from build123d import *

# Parameters (mm, degrees)
SKETCH_1_W          = 228
SKETCH_1_H          = 84
SKETCH_1_R          = 2.15
EXTRUDE_1_DEPTH     = 1
SKETCH_3_R          = 1.7
SKETCH_3_R_2        = 1.6
SKETCH_3_R_3        = 4
CUT_EXTRUDE_1_DEPTH = 10
SKETCH_4_R          = 3.5
SKETCH_4_R_2        = 1.6
CUT_EXTRUDE_2_DEPTH = 1
SKETCH_5_R          = 1.7
SKETCH_5_R_2        = 3
CUT_EXTRUDE_3_DEPTH = 10


with BuildPart() as part:
    # Эскиз1 → Вытянуть1 (new body)
    with BuildSketch(Plane.XY):
        Rectangle(SKETCH_1_W, SKETCH_1_H)
        with Locations((107, 32)):
            Circle(SKETCH_1_R, mode=Mode.SUBTRACT)
        with Locations(Location((-107, 32, 0), (0, 0, 180))):
            Circle(SKETCH_1_R, mode=Mode.SUBTRACT)
        with Locations((-107, -32)):
            Circle(SKETCH_1_R, mode=Mode.SUBTRACT)
        with Locations(Location((107, -32, 0), (0, 0, 180))):
            Circle(SKETCH_1_R, mode=Mode.SUBTRACT)
    extrude(amount=EXTRUDE_1_DEPTH)

    # Эскиз3 → Вырез-Вытянуть1 (cut)
    with BuildSketch(Plane.XY.offset(1)):
        with Locations((37, -22)):
            Circle(SKETCH_3_R)
        with Locations((84, -22)):
            Circle(SKETCH_3_R)
        with Locations((38.5, 17)):
            Circle(SKETCH_3_R_2)
        with Locations((82.5, 17)):
            Circle(SKETCH_3_R_2)
        with Locations((51.5, 22)):
            Circle(SKETCH_3_R_3)
        with Locations((69.5, 22)):
            Circle(SKETCH_3_R_3)
        with BuildLine():
            Line((40.14870942, -25.864196381), (40.875982147, -17.864196381))
            ThreePointArc((40.875982147, -17.864196381), (41.358314525, -16.892366164), (42.369821957, -16.5))
            Line((42.369821957, -16.5), (78.630178043, -16.5))
            ThreePointArc((78.630178043, -16.5), (79.641685475, -16.892366164), (80.124017853, -17.864196381))
            Line((80.124017853, -17.864196381), (80.85129058, -25.864196381))
            ThreePointArc((80.85129058, -25.864196381), (80.465084606, -27.011507432), (79.35745077, -27.5))
            Line((79.35745077, -27.5), (41.64254923, -27.5))
            ThreePointArc((41.64254923, -27.5), (40.534915394, -27.011507432), (40.14870942, -25.864196381))
        make_face()
    extrude(amount=-CUT_EXTRUDE_1_DEPTH, mode=Mode.SUBTRACT)

    # Эскиз4 → Вырез-Вытянуть2 (cut)
    with BuildSketch(Plane.XY.offset(1)):
        with Locations((-108, 9)):
            Circle(SKETCH_4_R)
        with Locations((-102, -15)):
            Circle(SKETCH_4_R_2)
        with Locations((-37, -15)):
            Circle(SKETCH_4_R_2)
        with Locations((-26, -15)):
            Circle(SKETCH_4_R_2)
        with Locations((23, -15)):
            Circle(SKETCH_4_R_2)
        with BuildLine():
            Line((-84.5, -9.5), (-54.5, -9.5))
            ThreePointArc((-54.5, -9.5), (-47, -17), (-54.5, -24.5))
            Line((-54.5, -24.5), (-84.5, -24.5))
            ThreePointArc((-84.5, -24.5), (-92, -17), (-84.5, -9.5))
        make_face()
        with BuildLine():
            Line((-9, -9.5), (6, -9.5))
            ThreePointArc((6, -9.5), (13.5, -17), (6, -24.5))
            Line((6, -24.5), (-9, -24.5))
            ThreePointArc((-9, -24.5), (-16.5, -17), (-9, -9.5))
        make_face()
    extrude(amount=-CUT_EXTRUDE_2_DEPTH, mode=Mode.SUBTRACT)

    # Эскиз5 → Вырез-Вытянуть3 (cut)
    with BuildSketch(Plane.XY.offset(1)):
        with Locations((-84, 22)):
            Circle(SKETCH_5_R)
        with Locations((6, 22)):
            Circle(SKETCH_5_R)
        with Locations((-4, 22)):
            Circle(SKETCH_5_R_2)
        with Locations((-14, 22)):
            Circle(SKETCH_5_R_2)
        with Locations((-24, 22)):
            Circle(SKETCH_5_R_2)
        with Locations((-34, 22)):
            Circle(SKETCH_5_R_2)
        with Locations((-44, 22)):
            Circle(SKETCH_5_R_2)
        with Locations((-54, 22)):
            Circle(SKETCH_5_R_2)
        with Locations((-64, 22)):
            Circle(SKETCH_5_R_2)
        with Locations((-74, 22)):
            Circle(SKETCH_5_R_2)
    extrude(amount=-CUT_EXTRUDE_3_DEPTH, mode=Mode.SUBTRACT)


solid = part.part
The model under review builds one solid part; all positions refer to its coordinate system, in mm. A direction names the side the tool comes from. Round coordinates to 2 decimals unless told otherwise and drop trailing zeros. Loops run counter-clockwise (first coordinate to the right, second up) from the corner with the lowest first, then second, coordinate; pieces in that order, holes last. Notation, with made-up numbers: (5, 50.25) -> (43, 50.25) arc R23 ccw to (43, 63.25) -> close; hole circle Ø5 at (50.25, 73.5). An arc over 180 degrees is marked (long way). One line per question, with ' | ' between items. Start each with the question number.
Item 1: Add section C-C, the plane x = -43. Write out the cut boundary in (y, z), then the cut area to 3 significant figures.
Item 2: Machinability: for faces 1 (the face through (-16.5, -17.16, 0.51)), 2 (the face through (-2, 1, 0)), which of the approach directions +Z, -Z, +X, -X, +Y, -Y give a long, thin tool a straight path to every point of the face, cutting with its end or side? Answer none if there is none.
Item 3: Add section B-B, the plane z = 0.8. Count the separate pieces of the cut face and the enclosed holes in it, then the cut area to 3 significant figures.
Item 4: Wall thickness on line 1 along Y through (x, z) = (107, 0.75); line 2 along Y through (x, z) = (-102, 0.7); line 3 along Y through (x, z) = (44, 0.55): over which ranges is each line inside the solid? List them lowest first. Write a range as [from, to].
Item 5: Add section A-A, the plane x = 51.5. Write out the cut boundary in (y, z), then the cut area to 3 significant figures.
Item 6: Draft analysis for pull direction X (two halves, no side actions). For faces 3 (the face through (13.5, -16.84, 0.51)), 4 (the face through (-2, 1, 1)), 5 (the face through (-66.4, 20.2, 0.5)), state which applies: +X half, -X half, draft (parallel to the pull), parting line (faces both ways), or undercut.
Return value:
1) outline: (-42, 0) -> (19.17, 0) -> (19.17, 1) -> (-42, 1) -> close; (24.83, 0) -> (42, 0) -> (42, 1) -> (24.83, 1) -> close | area: 78.3 mm2
2) face 1: +Z, -Z | face 2: -Z, +X, -X, +Y, -Y
3) separate pieces: 1 | enclosed holes: 28 | area: 17,200 mm2
4) line 1: y = [-42, -34.15], [-29.85, 29.85], [34.15, 42] | line 2: y = [-42, -16.6], [-13.4, 42] | line 3: y = [-42, -27.5], [-16.5, 42]
5) outline: (-42, 0) -> (-27.5, 0) -> (-27.5, 1) -> (-42, 1) -> close; (-16.5, 0) -> (18, 0) -> (18, 1) -> (-16.5, 1) -> close; (26, 0) -> (42, 0) -> (42, 1) -> (26, 1) -> close | area: 65.0 mm2
6) face 3: undercut | face 4: draft | face 5: undercut
